Model file for the job. Use its own axes, mm. Face numbers are marked on the shaded views. A direction names the side the tool comes from. Round coordinates to 2 decimals unless told otherwise and drop trailing zeros. Order: outer loops, then holes, each group sorted by start corner. A loop starts at its lowest first (then second) coordinate and runs counter-clockwise, first axis right, second up. Notation, with made-up numbers: (89, -24.75) - (135, -24.75) arc R28 cw to (135, 14.25) - close; hole circle Ø8 at (4.5, 55.5). An arc over 180 degrees is marked (long way). Put each result on its own line as item: value. Start each with the question number.
Item 1: Probe probe 1 along Z at (x, y) = (-10, 2.2); probe 2 along Z at (x, y) = (10, 1.1); probe 3 along Z at (x, y) = (0, 4.2). List the from-to ranges inside material, lowest first.
Item 2: Saw through at B-B on z = -10. List the corners of the cut face in (x, y), plus the area to 3 significant figures.
Item 3: Saw through at C-C on y = 2.3. List the corners of the cut face in (x, z), plus the area to 3 significant figures.
Item 4: Saw through at A-A on x = -8. List the corners of the cut face in (y, z), plus the area to 3 significant figures.
Item 5: Pin check, flat tips, straight feed: pin 1 Ø1 at (y, z) = (3, 18.5) entering from -X; pin 2 Ø2 at (x, y) = (19.5, 1.5) entering from +Z; pin 3 Ø3 at (x, y) = (15, 2) entering from -Z; pin 4 Ø3.5 at (x, z) = (10, 10) entering from +Y. Stop position of each tip, or through.
Item 6: Saw through at D-D on x = 0. List the corners of the cut face in (y, z).
Item 7: Which spindle directions (+Z, -Z, +X, -X, +Y, -Y) get a long thin tool onto all of the face, cutting with end or side? Do the marked faces 1 and 2. Say none if no direction does.
Autodesk Fusion 360 part; units mm, degrees
sketch "草图1" plane through (0, 0, 0) normal (0, 1, 0) x (1, 0, 0)
  circle A0 centre (0, 0) radius 25
extrude "拉伸1" add sketch "草图1" along normal blind 5
sketch "草图2" plane through (0, 5, 0) normal (0, 1, 0) x (-1, 0, 0)
  circle A0 centre (0, 0) radius 25
  circle A1 centre (0, 0) radius 20
extrude "拉伸2" cut sketch "草图2" against normal blind 2 contours A1
sketch "草图3" plane through (0, 3, 0) normal (0, 1, 0) x (-1, 0, 0)
  circle A0 centre (0, 0) radius 20
  circle A1 centre (7.861, -8.3613) radius 4.4141
cylinder "圆柱体基本要素1" cut diameter 6 height -10 placed x (1, 0, 0) y (0, 0, -1) z (0, 1, 0) at (-10, 3, -10)
cylinder "圆柱体基本要素2" cut diameter 6 height -8 placed x (1, 0, 0) y (0, 0, -1) z (0, 1, 0) at (10, 3, -10)
cylinder "圆柱体基本要素3" cut diameter 6 height -6 placed x (1, 0, 0) y (0, 0, -1) z (0, 1, 0) at (-10, 3, 10)
cylinder "圆柱体基本要素4" cut diameter 6 height -5 placed x (1, 0, 0) y (0, 0, -1) z (0, 1, 0) at (10, 3, 10)
extrude "拉伸3" cut sketch "草图3" against normal blind 5 contours A1
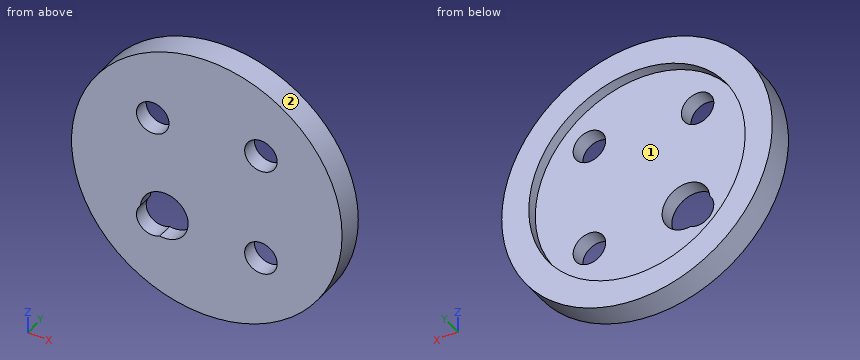
Results found:
1. probe 1: z = -22.91 to -13, -4.5 to 7, 13 to 22.91
1. probe 2: z = -22.91 to -13, -7 to 7, 13 to 22.91
1. probe 3: z = -25 to -20, 20 to 25
2. outline: (-22.91, 0) - (-13, 0) - (-13, 3) - (-17.32, 3) - (-17.32, 5) - (-22.91, 5) - close; (-3.76, 0) - (7, 0) - (7, 3) - (-3.76, 3) - close; (13, 0) - (22.91, 0) - (22.91, 5) - (17.32, 5) - (17.32, 3) - (13, 3) - close
2. area: 114 mm²
3. outline: circle Ø50 at (0, 0); hole circle Ø6 at (-10, 10); hole (-12.26, -8.03) arc R3 ccw to (-8.69, -12.7) arc R4.41 ccw (long way) to start; hole circle Ø6 at (10, -10); hole circle Ø6 at (10, 10)
3. area: 1,810 mm²
4. outline: (0, -23.69) - (5, -23.69) - (5, -18.33) - (3, -18.33) - (3, -12.77) - (0, -12.77) - close; (0, -3.95) - (3, -3.95) - (3, 7.76) - (0, 7.76) - close; (0, 12.24) - (3, 12.24) - (3, 18.33) - (5, 18.33) - (5, 23.69) - (0, 23.69) - close
4. area: 124 mm²
5. pin 1: stops at x = -17.35
5. pin 2: stops at z = 16.82
5. pin 3: stops at z = -21.04
5. pin 4: passes through
6. outline: (0, -25) - (5, -25) - (5, -20) - (3, -20) - (3, 20) - (5, 20) - (5, 25) - (0, 25) - close
7. face 1: +Y
7. face 2: +Y, -Y
